Geometry: see drawing. Coordinates: mm, zero at the bounding-box minimum. A direction names the side the tool comes from. Give positions to 0.01 mm unless a question says otherwise; leave off trailing zeros. Loops run counter-clockwise (first coordinate to the right, second up) from the corner with the lowest first, then second, coordinate; pieces in that order, holes last. Notation, with made-up numbers: M 27.25,72 L 68.25,72 A22 ccw 68.25,110 Z; hole C 71,15 d6. An arc over 180 degrees is marked long. Put each result on its own line as item: value.
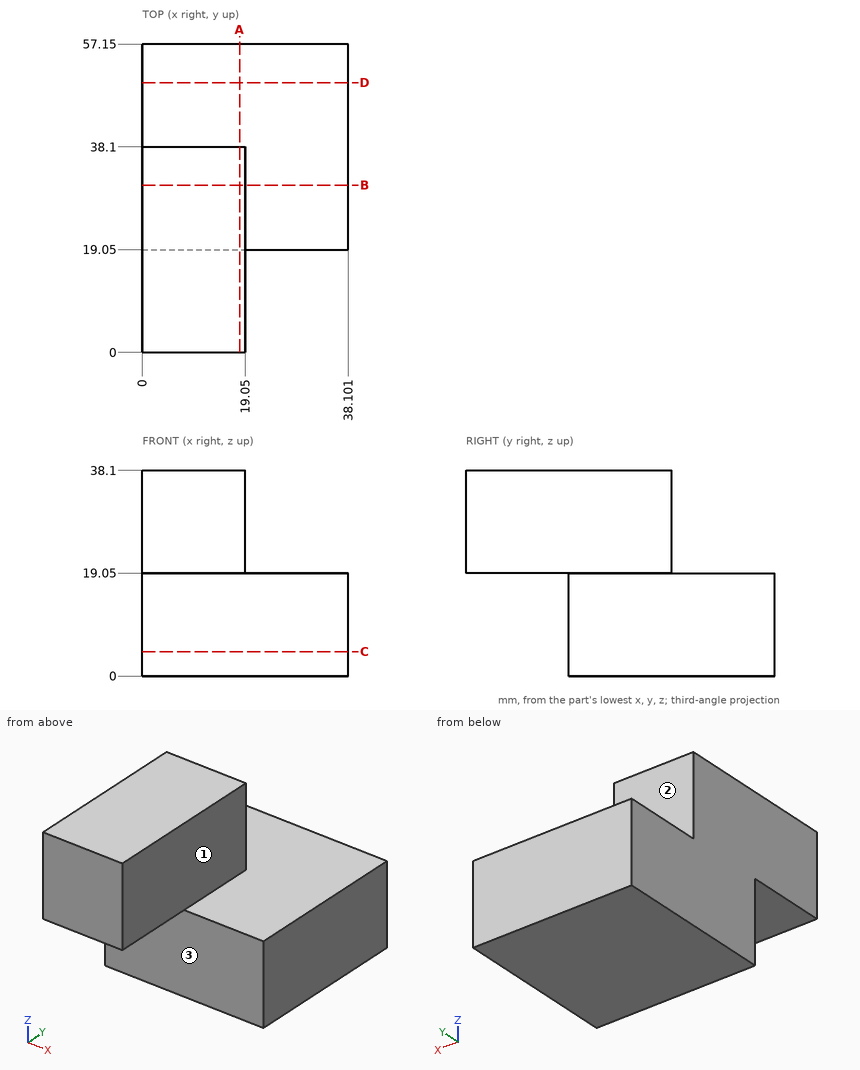
1. Section query A-A (x = 18). Output: boundary loops of the cut face in (y, z).
Found:
outline: M 0,19.05 L 19.05,19.05 L 19.05,0 L 57.15,0 L 57.15,19.05 L 38.1,19.05 L 38.1,38.1 L 0,38.1 Z
2. Section query D-D (y = 50). Output: boundary loops of the cut face in (x, z).
Found:
outline: M 0,0 L 38.1,0 L 38.1,19.05 L 0,19.05 Z
3. Material intervals for line 1 (Z direction, x = 31.5, y = 50.5); line 2 (Y direction, x = 16.5, z = 25), sorted ascending. Write a range as from..to.
Found:
line 1: 0..19.05
line 2: 0..38.1
4. Contact query for flat-ended pins moving along their axis: P1, Ø15, axis at x = 6, y = 6, coming from the -Z side; P2, Ø11.5, axis at x = 18.5, y = 45, coming from the +Z side; P3, Ø9.5, axis at y = 11, z = 26, coming from the +X side; P4, Ø2, axis at x = 22.5, z = 22, coming from the +Y side. Output: stop coordinate, or through.
Found:
P1: z = 19.05
P2: z = 19.05
P3: x = 19.05
P4: through
5. Access query for the marked faces 1, 2 and 3. Directions: +Z, -Z, +X, -X, +Y, -Y. A direction counts if a zero-diameter tool reaches every point of the face in a straight line with its end or side. Return the directions, or none.
Found:
face 1: +Z, +X, +Y, -Y
face 2: +Z, +X, -X, +Y
face 3: -Z, +X, -X, -Y
6. Section query C-C (z = 4.5). Output: boundary loops of the cut face in (x, y), plus the area to 3 significant figures.
Found:
outline: M 0,19.05 L 38.1,19.05 L 38.1,57.15 L 0,57.15 Z
area: 1,450 mm^2
7. Section query B-B (y = 31). Output: boundary loops of the cut face in (x, z).
Found:
outline: M 0,0 L 38.1,0 L 38.1,19.05 L 19.05,19.05 L 19.05,38.1 L 0,38.1 Z
